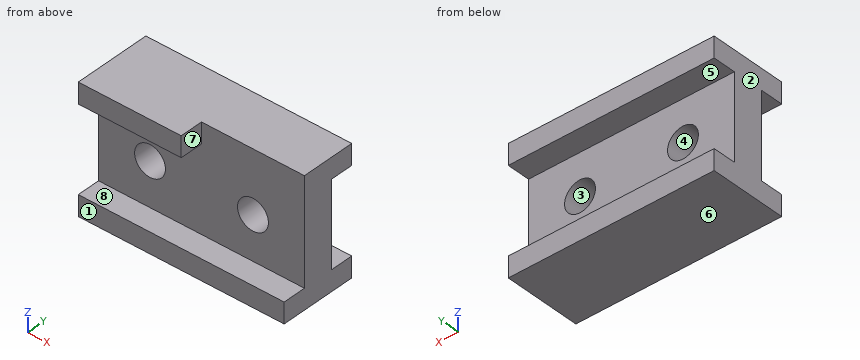
```python
from build123d import *

# Parameters (mm, degrees)
F1_DEPTH = 254
F2_R     = 19.05
F3_DEPTH = 101.346
F2_W     = 127
F2_H     = 25.4
F4_DEPTH = 28.575


with BuildPart() as f1:
    # F0 (on Right) → F1 (new body)
    with BuildSketch(Plane.YZ):
        Polygon((0, 25.4), (0, 0), (95.25, 0), (95.25, 25.4), (66.675, 25.4), (66.675, 130.175), (95.25, 130.175), (95.25, 155.575), (28.575, 155.575), (28.575, 25.4), align=None)
    extrude(amount=F1_DEPTH)

    # F2 (on face) → F3 (cut)
    with BuildSketch(Plane.XZ.offset(-28.575)):
        with Locations((63.5, 79.375)):
            Circle(F2_R)
        with Locations((190.5, 79.375)):
            Circle(F2_R)
    extrude(amount=-F3_DEPTH, mode=Mode.SUBTRACT)

    # F2 (on face) → F4 (join, through all)
    with BuildSketch(Plane.XZ.offset(-28.575)):
        with Locations((63.5, 142.875)):
            Rectangle(F2_W, F2_H)
    extrude(amount=F4_DEPTH)


solid = f1.part
```
Source: CAD feature listing. Evaluate the final solid. Frame: model axes, mm. Face numbers are marked on the shaded views. A direction names the side the tool comes from. Give positions to 0.01 mm unless a question says otherwise; leave off trailing zeros. Write each loop counter-clockwise with the first axis right and the second up, starting at its lowest first coordinate (ties: lowest second). Pieces come first, ordered by that corner, then holes. Notation, with made-up numbers: (17.25, -8.75) - (38.25, -8.75) arc R17 cw to (38.25, 6.25) - close; hole circle Ø6 at (-8.75, 56). An arc over 180 degrees is marked (long way). One line per item, written item: value. Start each with the question number.
Q1. Section query A-A, the plane x = 190.5. Return the cut outline in (y, z) (3 decimals).
Q2. Section query B-B, the plane x = 218. Return the cut outline in (y, z) (3 decimals), then the cut area to 3 significant figures.
Q3. First-contact query: pin 1 Ø4 at (x, z) = (46.5, 49.5) entering from -Y (3 decimals); pin 2 Ø10 at (x, z) = (82, 47) entering from +Y (3 decimals). Flat tips, straight axial feed; report the tip coordinate or a pass-through.
Q4. Section query D-D, the plane y = 33.5. Return the cut outline in (x, z) (3 decimals), then the cut area to 3 significant figures.
Q5. Section query C-C, the plane z = 75. Return the cut outline in (x, y) (3 decimals).
Q6. Material intervals for probe 1 along Z at (x, y) = (229.5, 73) (3 decimals); probe 2 along Z at (x, y) = (190.5, 54) (3 decimals); probe 3 along Z at (x, y) = (225, 20), sorted ascending. Write a range as from..to.
Q7. Set-up query: the marked faces 5, 6, 7 and 8. Return all of +Z, -Z, +X, -X, +Y, -Y with unobstructed straight access to the full face (end or side cutting, diameter ignored); none if empty.
Q8. Draft query along X for the marked faces 1, 2, 3 and 4. Return one class per face: +X half, -X half, draft (parallel to the pull), parting line (faces both ways), or undercut.
Answer:
1. outline: (0, 0) - (95.25, 0) - (95.25, 25.4) - (66.675, 25.4) - (66.675, 60.325) - (28.575, 60.325) - (28.575, 25.4) - (0, 25.4) - close; (28.575, 98.425) - (66.675, 98.425) - (66.675, 130.175) - (95.25, 130.175) - (95.25, 155.575) - (28.575, 155.575) - close
2. outline: (0, 0) - (95.25, 0) - (95.25, 25.4) - (66.675, 25.4) - (66.675, 130.175) - (95.25, 130.175) - (95.25, 155.575) - (28.575, 155.575) - (28.575, 25.4) - (0, 25.4) - close
2. area: 8,100 mm2
3. pin 1: stops at y = 28.575
3. pin 2: stops at y = 66.675
4. outline: (0, 0) - (254, 0) - (254, 155.575) - (0, 155.575) - close; hole circle Ø38.1 at (63.5, 79.375); hole circle Ø38.1 at (190.5, 79.375)
4. area: 37,200 mm2
5. outline: (0, 28.575) - (44.959, 28.575) - (44.959, 66.675) - (0, 66.675) - close; (82.041, 28.575) - (171.959, 28.575) - (171.959, 66.675) - (82.041, 66.675) - close; (209.041, 28.575) - (254, 28.575) - (254, 66.675) - (209.041, 66.675) - close
6. probe 1: z = 0..25.4, 130.175..155.575
6. probe 2: z = 0..60.325, 98.425..155.575
6. probe 3: z = 0..25.4
7. face 5: +X, -X, +Y
7. face 6: -Z, +X, -X, +Y, -Y
7. face 7: +Z, +X, -Y
7. face 8: +X, -X, -Y
8. face 1: draft
8. face 2: -X half
8. face 3: undercut
8. face 4: undercut
